from build123d import *

# Parameters (mm, degrees)
SKETCH_1_W                    = 4.65
SKETCH_1_H                    = 8.6
EXTRUDE_1_DEPTH               = 4
EXTRUDE_2_DEPTH               = 4
CUT_EXTRUDE_1_DEPTH           = 3.5
PATTERN_LINEAR_4_COUNT        = 7
PATTERN_LINEAR_4_PITCH        = 4.65
PATTERN_LINEAR_4_COPY_1_DEPTH = 4
PATTERN_LINEAR_4_COPY_2_DEPTH = 4
PATTERN_LINEAR_4_COPY_3_DEPTH = 4
PATTERN_LINEAR_4_COPY_4_DEPTH = 4
PATTERN_LINEAR_4_COPY_5_DEPTH = 4
PATTERN_LINEAR_4_COPY_6_DEPTH = 4
EXTRUDE_START                 = 1
EXTRUDE_4_DEPTH               = 25.9
FILLET_1_R                    = 0.1


with BuildPart() as part:
    # 草图1 → 凸台-拉伸1 (new body)
    with BuildSketch(Plane(origin=(0, 0, 0), x_dir=(1, 0, 0), z_dir=(0, 1, 0))):
        Rectangle(SKETCH_1_W, SKETCH_1_H)
    extrude_1 = extrude(amount=EXTRUDE_1_DEPTH)

    # 草图3 → 凸台-拉伸2 (add)
    with BuildSketch(Plane(origin=(0, 0, 0), x_dir=(1, 0, 0), z_dir=(0, 1, 0))):
        Polygon((0.625, 7.5), (-0.625, 7.5), (-1.7, 4.3), (1.7, 4.3), align=None)
    extrude_2 = extrude(amount=EXTRUDE_2_DEPTH)

    # 镜向1: 凸台-拉伸2 across plane
    add(extrude_2.mirror(Plane.XY))

    # 草图4 → 切除-拉伸1 (cut, symmetric)
    with BuildSketch(Plane.XY):
        Polygon((-0.625, 4), (-2.325, 4), (-2.325, 0.8), (-1.7, 0.8), align=None)
        Polygon((1.7, 0.8), (2.325, 0.8), (2.325, 4), (0.625, 4), align=None)
    cut_extrude_1 = extrude(amount=CUT_EXTRUDE_1_DEPTH, both=True, mode=Mode.SUBTRACT)

    # 阵列(线性)4: 凸台-拉伸1, 凸台-拉伸2, 切除-拉伸1 ×7
    with Locations(*[(i * PATTERN_LINEAR_4_PITCH, 0, 0) for i in range(1, PATTERN_LINEAR_4_COUNT)]):
        add(extrude_1)
        add(extrude_2)
        add(cut_extrude_1, mode=Mode.SUBTRACT)

    # 阵列(线性)4 copy 1 sketch → 阵列(线性)4 copy 1 (add)
    with BuildSketch(Plane(origin=(4.65, 0, 0), x_dir=(1, 0, 0), z_dir=(0, 1, 0))):
        Polygon((0.625, -7.5), (-0.625, -7.5), (-1.7, -4.3), (1.7, -4.3), align=None)
    extrude(amount=PATTERN_LINEAR_4_COPY_1_DEPTH)

    # 阵列(线性)4 copy 2 sketch → 阵列(线性)4 copy 2 (add)
    with BuildSketch(Plane(origin=(9.3, 0, 0), x_dir=(1, 0, 0), z_dir=(0, 1, 0))):
        Polygon((0.625, -7.5), (-0.625, -7.5), (-1.7, -4.3), (1.7, -4.3), align=None)
    extrude(amount=PATTERN_LINEAR_4_COPY_2_DEPTH)

    # 阵列(线性)4 copy 3 sketch → 阵列(线性)4 copy 3 (add)
    with BuildSketch(Plane(origin=(13.95, 0, 0), x_dir=(1, 0, 0), z_dir=(0, 1, 0))):
        Polygon((0.625, -7.5), (-0.625, -7.5), (-1.7, -4.3), (1.7, -4.3), align=None)
    extrude(amount=PATTERN_LINEAR_4_COPY_3_DEPTH)

    # 阵列(线性)4 copy 4 sketch → 阵列(线性)4 copy 4 (add)
    with BuildSketch(Plane(origin=(18.6, 0, 0), x_dir=(1, 0, 0), z_dir=(0, 1, 0))):
        Polygon((0.625, -7.5), (-0.625, -7.5), (-1.7, -4.3), (1.7, -4.3), align=None)
    extrude(amount=PATTERN_LINEAR_4_COPY_4_DEPTH)

    # 阵列(线性)4 copy 5 sketch → 阵列(线性)4 copy 5 (add)
    with BuildSketch(Plane(origin=(23.25, 0, 0), x_dir=(1, 0, 0), z_dir=(0, 1, 0))):
        Polygon((0.625, -7.5), (-0.625, -7.5), (-1.7, -4.3), (1.7, -4.3), align=None)
    extrude(amount=PATTERN_LINEAR_4_COPY_5_DEPTH)

    # 阵列(线性)4 copy 6 sketch → 阵列(线性)4 copy 6 (add)
    with BuildSketch(Plane(origin=(27.9, 0, 0), x_dir=(1, 0, 0), z_dir=(0, 1, 0))):
        Polygon((0.625, -7.5), (-0.625, -7.5), (-1.7, -4.3), (1.7, -4.3), align=None)
    extrude(amount=PATTERN_LINEAR_4_COPY_6_DEPTH)

    # 草图6 → 凸台-拉伸4 (add)
    with BuildSketch(Plane(origin=(0, 0, 0), x_dir=(0, 0, -1), z_dir=(1, 0, 0)).offset(EXTRUDE_START)):
        with BuildLine():
            Line((1.5, 0), (0.5, 0))
            Line((0.5, 0), (0.5, -1.07225346))
            Line((0.5, -1.07225346), (1.165769145, -2.5))
            Line((1.165769145, -2.5), (1.95, -2.5))
            Line((1.95, -2.5), (1.95, -1.555590279))
            ThreePointArc((1.95, -1.555590279), (1.780042303, -1.088161527), (1.5, -0.677124344))
            Line((1.5, -0.677124344), (1.5, 0))
        make_face()
        with BuildLine():
            Line((-0.5, -1.07225346), (-1.165769145, -2.5))
            Line((-1.165769145, -2.5), (-1.95, -2.5))
            Line((-1.95, -2.5), (-1.95, -1.555590279))
            ThreePointArc((-1.95, -1.555590279), (-1.780042303, -1.088161527), (-1.5, -0.677124344))
            Line((-1.5, -0.677124344), (-1.5, 0))
            Line((-1.5, 0), (-0.5, 0))
            Line((-0.5, 0), (-0.5, -1.07225346))
        make_face()
    extrude(amount=EXTRUDE_4_DEPTH)

    # 圆角1
    fillet_1_edges = [part.edges().sort_by_distance(p)[0] for p in [
        (1, -2.5, -1.557884573),
        (13.95, -2.5, -1.165769145),
        (13.95, -2.5, -1.95),
        (26.9, -2.5, -1.557884573),
        (1, -2.5, 1.557884573),
        (13.95, -2.5, 1.95),
        (13.95, -2.5, 1.165769145),
        (26.9, -2.5, 1.557884573),
    ]]
    fillet(fillet_1_edges, radius=FILLET_1_R)


solid = part.part
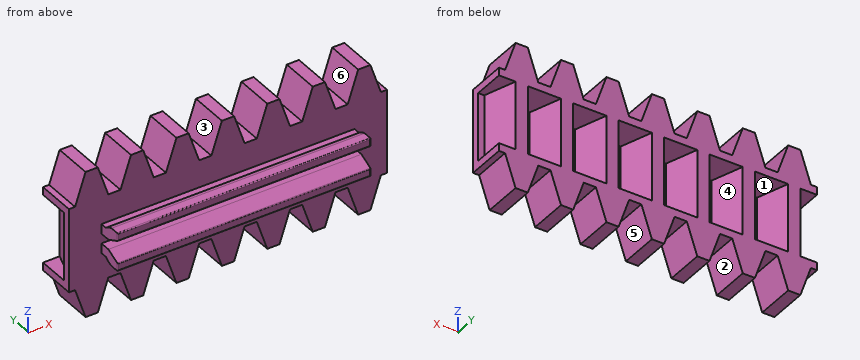
Geometry check sheet. Reference: the model listing, model coordinates, mm. Face numbers are marked on the shaded views. A direction names the side the tool comes from. Give positions to 0.01 mm unless a question says otherwise; leave off trailing zeros. Loops run counter-clockwise (first coordinate to the right, second up) from the corner with the lowest first, then second, coordinate; pieces in that order, holes last. Notation, with made-up numbers: (86, -38.75) -> (134, -38.75) arc R7 ccw to (134, -28.75) -> close; hole circle Ø9 at (-34.75, 3.25). An arc over 180 degrees is marked (long way). Answer in a Markdown table with one row per item. Add a question column.
1) Cross-section at B-B on x = 4.5. Record the boundary of the cut face in (y, z), and give its area (3 significant figures).
2) Gauge pin test, flat ends, axial feed: P1, Ø0.5, axis at x = 10, y = 0, coming from the +Z side; P2, Ø0.7, axis at y = -1.5, z = 1, coming from the -X side; P3, Ø4, axis at x = 21.5, z = -4.5, coming from the -Y side; P4, Ø0.5, axis at x = 8, y = -0.5, coming from the -Z side. Record the tip position at first contact, or that the pin passes through.
3) Cross-section at A-A on z = 6.75. Record the boundary of the cut face in (x, y).
4) Draft check along Z on the marked faces 1, 2 and 3. Enter one of: pulls with the +Z half, pulls with the -Z half, needs draft (parallel to the pull), parting line crosses it, or undercut.
5) Set-up check for the marked faces 4, 5 and 6: record each of +Z, -Z, +X, -X, +Y, -Y from which the full face is reachable in a straight line by a thin tool's end or side.
6) Material ranges on probe 1 along Z at (x, y) = (7, 3.25); probe 2 along X at (y, z) = (-1, -1); probe 3 along Y at (x, z) = (15, 6), recorded low to high. Write a range as from..to.
7) Cross-section at D-D on y = 2.25. State how many separate pieces and enclosed holes the cut face has, and give its area (3 significant figures).
8) Cross-section at C-C on z = -6.5. Record the boundary of the cut face in (x, y).
Outcome:
| question | item | result |
|---|---|---|
| 1 | outline | (-2.5, -1.85) arc R0.1 ccw to (-2.4, -1.95) -> (-1.56, -1.95) arc R2 ccw to (-0.68, -1.5) -> (0, -1.5) -> (0, -7.5) -> (4, -7.5) -> (4, 7.5) -> (0, 7.5) -> (0, 1.5) -> (-0.68, 1.5) arc R2 ccw to (-1.56, 1.95) -> (-2.4, 1.95) arc R0.1 ccw to (-2.5, 1.85) -> (-2.5, 1.23) arc R0.1 ccw to (-2.44, 1.14) -> (-1.07, 0.5) -> (0, 0.5) -> (0, -0.5) -> (-1.07, -0.5) -> (-2.44, -1.14) arc R0.1 ccw to (-2.5, -1.23) -> close |
| 1 | area | 65.4 mm^2 |
| 2 | P1 | stops at z = 7.5 |
| 2 | P2 | stops at x = 1 |
| 2 | P3 | stops at y = 0 |
| 2 | P4 | stops at z = -1.56 |
| 3 | outline | (-0.88, 0) -> (0.88, 0) -> (0.88, 4) -> (-0.88, 4) -> close; (3.77, 0) -> (5.53, 0) -> (5.53, 4) -> (3.77, 4) -> close; (8.42, 0) -> (10.18, 0) -> (10.18, 4) -> (8.42, 4) -> close; (13.07, 0) -> (14.83, 0) -> (14.83, 4) -> (13.07, 4) -> close; (17.72, 0) -> (19.48, 0) -> (19.48, 4) -> (17.72, 4) -> close; (22.37, 0) -> (24.13, 0) -> (24.13, 4) -> (22.37, 4) -> close; (27.02, 0) -> (28.78, 0) -> (28.78, 4) -> (27.02, 4) -> close |
| 4 | face 1 | undercut |
| 4 | face 2 | pulls with the -Z half |
| 4 | face 3 | pulls with the +Z half |
| 5 | face 4 | +Y |
| 5 | face 5 | -Z, +Y, -Y |
| 5 | face 6 | +Z, +Y, -Y |
| 6 | probe 1 | z = -4.3..-3.5, 3.5..4.3 |
| 6 | probe 2 | x = 1..26.9 |
| 6 | probe 3 | y = 0..4 |
| 7 | separate pieces | 1 |
| 7 | enclosed holes | 6 |
| 7 | area | 275 mm^2 |
| 8 | outline | (-0.96, 0) -> (0.96, 0) -> (0.96, 4) -> (-0.96, 4) -> close; (3.69, 0) -> (5.61, 0) -> (5.61, 4) -> (3.69, 4) -> close; (8.34, 0) -> (10.26, 0) -> (10.26, 4) -> (8.34, 4) -> close; (12.99, 0) -> (14.91, 0) -> (14.91, 4) -> (12.99, 4) -> close; (17.64, 0) -> (19.56, 0) -> (19.56, 4) -> (17.64, 4) -> close; (22.29, 0) -> (24.21, 0) -> (24.21, 4) -> (22.29, 4) -> close; (26.94, 0) -> (28.86, 0) -> (28.86, 4) -> (26.94, 4) -> close |
